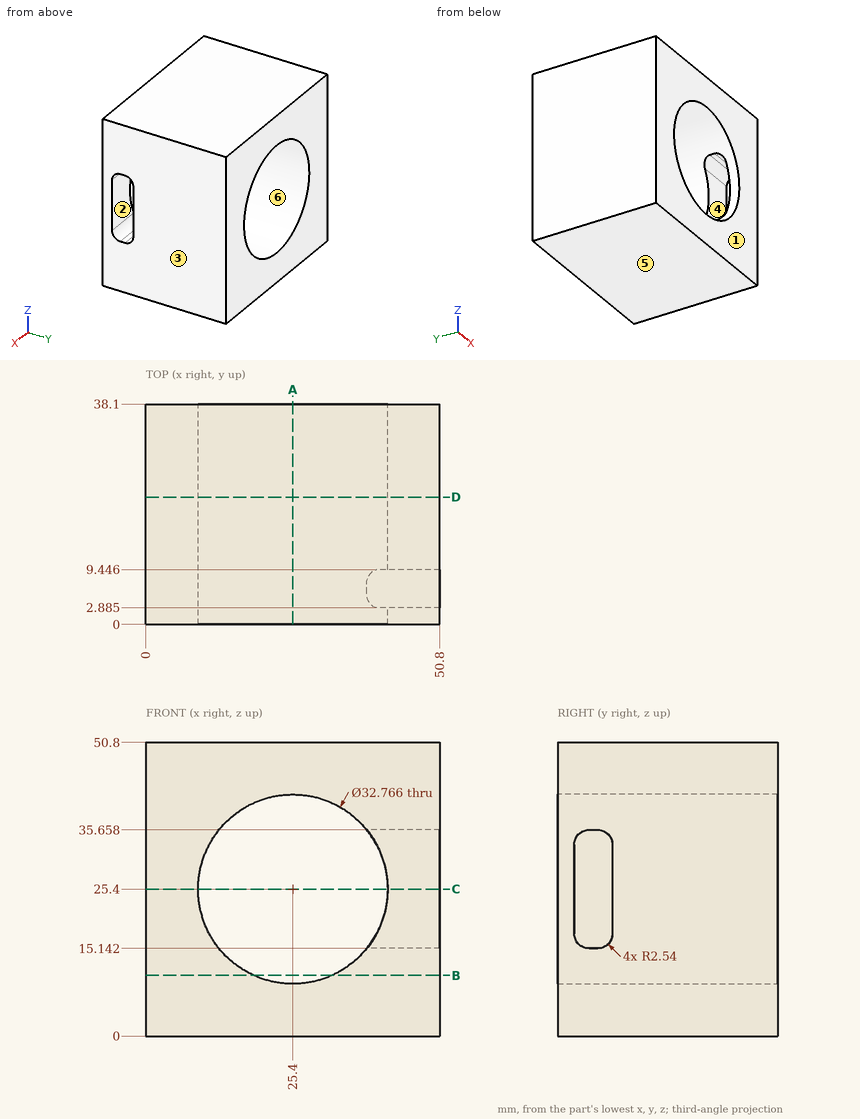
Study the drawing (mm; zero at the part's minimum x, y, z) and answer. A direction names the side the tool comes from. Round coordinates to 2 decimals unless told otherwise and drop trailing zeros. Write each loop counter-clockwise with the first axis right and the second up, starting at its lowest first coordinate (ties: lowest second). Pieces come first, ordered by that corner, then holes.
1) A cutting plane is placed at D-D (y = 22). Give the vertices of the cut face in (x, z), plus the area to 3 significant figures.
2) Given pin 1 Ø8 at (x, z) = (35.5, 22.5) entering from -Y, flat-ended and moving along its own axis, determine where the tip first touches the part or whether it passes through.
3) A tool of negligible diameter and unlimited length cuts with its end or side. For the marked faces 1 and 2, from which of +Z, -Z, +X, -X, +Y, -Y can it reach the whole face along a straight path? Write none if from no direction.
4) Straight lines are drawn through the part: line 1 (Z direction, x = 25, y = 29); line 2 (Z direction, x = 23.5, y = 23). For each, find the intervals that lie inside material, in ascending order.
5) A cutting plane is placed at B-B (z = 10.5). Give the vertices of the cut face in (x, y), plus the area to 3 significant figures.
6) A cutting plane is placed at A-A (x = 25.4). Give the vertices of the cut face in (y, z), plus the area to 3 significant figures.
7) The mould has two halves that part along Z. Classify the marked faces 3, 4, 5 and 6: pulls with the +Z half, pulls with the -Z half, needs draft (parallel to the pull), parting line crosses it, or undercut.
8) A cutting plane is placed at C-C (z = 25.4). Give the vertices of the cut face in (x, y) (1 decimal), plus the area to 3 significant figures.
Completed:
1. outline: (0, 0) - (50.8, 0) - (50.8, 50.8) - (0, 50.8) - close; hole circle Ø32.77 at (25.4, 25.4)
1. area: 1,740 mm2
2. pin 1: passes through
3. face 1: +Z, -Z, +X, -X, -Y
3. face 2: +X
4. line 1: z = 0 to 9.02, 41.78 to 50.8
4. line 2: z = 0 to 9.13, 41.67 to 50.8
5. outline: (0, 0) - (18.59, 0) - (18.59, 38.1) - (0, 38.1) - close; (32.21, 0) - (50.8, 0) - (50.8, 38.1) - (32.21, 38.1) - close
5. area: 1,420 mm2
6. outline: (0, 0) - (38.1, 0) - (38.1, 9.02) - (0, 9.02) - close; (0, 41.78) - (38.1, 41.78) - (38.1, 50.8) - (0, 50.8) - close
6. area: 687 mm2
7. face 3: needs draft
7. face 4: undercut
7. face 5: pulls with the -Z half
7. face 6: undercut
8. outline: (0, 0) - (9, 0) - (9, 38.1) - (0, 38.1) - close; (41.8, 0) - (50.8, 0) - (50.8, 2.9) - (41.8, 2.9) - close; (41.8, 9.4) - (50.8, 9.4) - (50.8, 38.1) - (41.8, 38.1) - close
8. area: 628 mm2
